```python
from build123d import *

# Parameters (mm, degrees)
SCHIZZO1_R                   = 4
SCHIZZO1_R_2                 = 2
ESTRUSIONE_ESTRUSIONE1_DEPTH = 5
SCHIZZO2_R                   = 2
TAGLIO_ESTRUSIONE1_DEPTH     = 10


with BuildPart() as part:
    # Schizzo1 → Estrusione-Estrusione1 (new body)
    with BuildSketch(Plane.XY):
        with BuildLine():
            ThreePointArc((-1.545685279, 7.338995641), (-7.37775549, -1.348600733), (1.150548918, -7.411223731))
            ThreePointArc((1.150548918, -7.411223731), (75.443261143, -2.885528453), (149.288277512, -12.20231786))
            ThreePointArc((149.288277512, -12.20231786), (152.870711747, -12.469637567), (156.381230514, -11.707041436))
            ThreePointArc((156.381230514, -11.707041436), (178.7761584, -6.547142951), (201.742232266, -7.393782545))
            ThreePointArc((201.742232266, -7.393782545), (210.367795627, -1.401994151), (204.545685279, 7.338995641))
            ThreePointArc((204.545685279, 7.338995641), (101.5, 18.072619578), (-1.545685279, 7.338995641))
        make_face()
        Circle(SCHIZZO1_R, mode=Mode.SUBTRACT)
        with Locations((203, 0)):
            Circle(SCHIZZO1_R_2, mode=Mode.SUBTRACT)
        with Locations((152, 0)):
            Circle(SCHIZZO1_R_2, mode=Mode.SUBTRACT)
    extrude(amount=ESTRUSIONE_ESTRUSIONE1_DEPTH)

    # Schizzo2 → Taglio-Estrusione1 (cut)
    with BuildSketch(Plane.XY.offset(5)):
        with Locations((21.792647349, 3.923925867)):
            Circle(SCHIZZO2_R)
        with Locations((115.643522851, 5.673925867)):
            Circle(SCHIZZO2_R)
        with Locations((180.602574062, 1.58663817)):
            Circle(SCHIZZO2_R)
    extrude(amount=-TAGLIO_ESTRUSIONE1_DEPTH, mode=Mode.SUBTRACT)


solid = part.part
```
Here's how the part is built. I have some questions about the finished solid (model axes, mm). Coordinates: 2 decimals unless noted, no trailing zeros. Loops run counter-clockwise (first coordinate to the right, second up) from the corner with the lowest first, then second, coordinate; pieces in that order, holes last. Notation, with made-up numbers: (0, 63) - (31, 63) arc R22 cw to (31, 74) - close; hole circle Ø3 at (36.25, 51.5). An arc over 180 degrees is marked (long way). Answer as CSV lines item,"result".
Q1. If we section it at A-A, the plane x = 152: Write out the boundary of the cut face in (y, z).
Response:
outline,"(-12.5, 0) - (-2, 0) - (-2, 5) - (-12.5, 5) - close; (2, 0) - (15.52, 0) - (15.52, 5) - (2, 5) - close"
Q2. For pin 1 (2 mm diameter, centred on x = 113.5, z = 2.5, fed in from -Y); pin 2 (1.5 mm diameter, centred on y = -5.5, z = 1, fed in from +X); pin 3 (2 mm diameter, centred on x = 130, z = 4, fed in from -Y), each with a flat end and sliding along its axis, tell me the tip position at first contact or that it passes through.
Response:
pin 1,"y = -6.07"
pin 2,"x = 208.8"
pin 3,"y = -8.58"
Q3. If I drill on L1, parallel to X at y = 4.5, z = 2.1; L2, parallel to X at y = -2.5, z = 2.95; L3, parallel to Y at x = 2.5, z = 0.75, over which ranges is the centre line in solid material (lowest first)? Write a range as [from, to].
Response:
L1,"[-6, 19.88], [23.71, 114.02], [117.26, 209]"
L2,"[-7.07, -3.12], [3.12, 210.07]"
L3,"[-7.2, -3.12], [3.12, 8.17]"
Q4. We'd pull the mould along Y, two halves only. Please class faces 1 (the face through (100, 3, 0)), 2 (the face through (150, 0, 2)), 3 (the face through (74.4, -2.853, 2.465)): pulls with the +Y half, pulls with the -Y half, needs draft (parallel to the pull), parting line crosses it, or undercut.
Response:
face 1,"needs draft"
face 2,"undercut"
face 3,"pulls with the -Y half"
Q5. If we section it at D-D, the plane x = 127.5: Write out the boundary of the cut face in (y, z), and give its area (3 significant figures).
Response:
outline,"(-7.99, 0) - (17.4, 0) - (17.4, 5) - (-7.99, 5) - close"
area,"127 mm2"
Q6. If we section it at C-C, the plane y = 11.5: Write out the boundary of the cut face in (x, z).
Response:
outline,"(20.7, 0) - (182.3, 0) - (182.3, 5) - (20.7, 5) - close"
Q7. If we section it at B-B, the plane z = 1.8: Write out the boundary of the cut face in (x, y), and give its area (3 significant figures).
Response:
outline,"(-1.55, 7.34) arc R7.5 ccw to (1.15, -7.41) arc R400 cw to (149.29, -12.2) arc R12.5 ccw to (156.38, -11.71) arc R87.54 cw to (201.74, -7.39) arc R7.5 ccw to (204.55, 7.34) arc R500 ccw to start; hole circle Ø8 at (0, 0); hole circle Ø4 at (21.79, 3.92); hole circle Ø4 at (115.64, 5.67); hole circle Ø4 at (152, 0); hole circle Ø4 at (180.6, 1.59); hole circle Ø4 at (203, 0)"
area,"4,240 mm2"
